```python
from build123d import *

# Parameters (mm, degrees)
SKETCH1_W           = 154.5
SKETCH1_H           = 74.4
BOSS_EXTRUDE1_DEPTH = 7.4
FILLET1_R           = 10
CHAMFER1_SIZE       = 1
FILLET2_R           = 2
SKETCH2_R           = 4.3
BOSS_EXTRUDE2_DEPTH = 0.6
CHAMFER2_SIZE       = 0.3
CUT_EXTRUDE1_DEPTH  = 6.75


with BuildPart() as part:
    # Sketch1 → Boss-Extrude1 (new body)
    with BuildSketch(Plane(origin=(0, 0, 0), x_dir=(1, 0, 0), z_dir=(0, 1, 0))):
        Rectangle(SKETCH1_W, SKETCH1_H)
    extrude(amount=BOSS_EXTRUDE1_DEPTH)

    # Fillet1
    fillet1_edges = [part.edges().sort_by_distance(p)[0] for p in [
        (77.25, 3.7, 37.2),
        (-77.25, 3.7, 37.2),
        (-77.25, 3.7, -37.2),
        (77.25, 3.7, -37.2),
    ]]
    fillet(fillet1_edges, radius=FILLET1_R)

    # Chamfer1
    chamfer1_edges = [part.edges().sort_by_distance(p)[0] for p in [
        (-77.25, 7.4, 0),
        (0, 7.4, -37.2),
        (77.25, 7.4, 0),
        (0, 7.4, 37.2),
        (74.321067812, 7.4, 34.271067812),
        (-74.321067812, 7.4, 34.271067812),
        (74.321067812, 7.4, -34.271067812),
        (-74.321067812, 7.4, -34.271067812),
    ]]
    chamfer(chamfer1_edges, length=CHAMFER1_SIZE)

    # Fillet2
    fillet2_edges = [part.edges().sort_by_distance(p)[0] for p in [
        (-77.25, 0, 0),
        (77.25, 0, 0),
        (0, 0, 37.2),
        (0, 0, -37.2),
        (74.321067812, 0, 34.271067812),
        (-74.321067812, 0, 34.271067812),
        (74.321067812, 0, -34.271067812),
        (-74.321067812, 0, -34.271067812),
    ]]
    fillet(fillet2_edges, radius=FILLET2_R)

    # Sketch2 → Boss-Extrude2 (add)
    with BuildSketch(Plane.XZ):
        with Locations((-68.95, -13.75)):
            Circle(SKETCH2_R)
        with BuildLine():
            Line((-73.25, -13.75), (-73.25, -23.65))
            ThreePointArc((-73.25, -23.65), (-68.95, -19.35), (-64.65, -23.65))
            Line((-64.65, -23.65), (-64.65, -13.75))
            ThreePointArc((-64.65, -13.75), (-68.95, -18.05), (-73.25, -13.75))
        make_face()
        with Locations((-68.95, -23.65)):
            Circle(SKETCH2_R)
    extrude(amount=BOSS_EXTRUDE2_DEPTH)

    # Chamfer2
    chamfer2_edges = [part.edges().sort_by_distance(p)[0] for p in [
        (-64.65, -0.6, -18.7),
        (-73.25, -0.6, -18.7),
        (-68.95, -0.6, -9.45),
        (-68.95, -0.6, -27.95),
    ]]
    chamfer(chamfer2_edges, length=CHAMFER2_SIZE)

    # Sketch3 → Cut-Extrude1 (cut)
    with BuildSketch(Plane(origin=(77.25, 0, 0), x_dir=(0, 0, -1), z_dir=(1, 0, 0))):
        with BuildLine():
            Line((-2.9, 4.8), (2.9, 4.8))
            ThreePointArc((2.9, 4.8), (4.2, 3.5), (2.9, 2.2))
            Line((2.9, 2.2), (-2.9, 2.2))
            ThreePointArc((-2.9, 2.2), (-4.2, 3.5), (-2.9, 4.8))
        make_face()
    extrude(amount=-CUT_EXTRUDE1_DEPTH, mode=Mode.SUBTRACT)


solid = part.part
```
The listing builds one solid part. Answer for the finished solid, in the listing's coordinates (mm). A direction names the side the tool comes from. Give positions to 0.01 mm unless a question says otherwise; leave off trailing zeros. Order: outer loops, then holes, each group sorted by start corner. A loop starts at its lowest first (then second) coordinate and runs counter-clockwise, first axis right, second up. Notation, with made-up numbers: (10.25, 53) -> (57.25, 53) arc R18 ccw to (57.25, 79) -> close; hole circle Ø11 at (-24.75, 56). An arc over 180 degrees is marked (long way). Answer as a JSON object with one key per item and string values. Group by question number.
Item 1: A tool of negligible diameter and unlimited length cuts with its end or side. For faces 4 (the flat face through (70.5, 4, 0)), 5 (the conical face through (-73.798, 7.24, -33.605)), from which of +Z, -Z, +X, -X, +Y, -Y can it reach the whole face along a straight path? Write none if from no direction.
Item 2: The part is cut by section B-B on x = -31.5. Write down the section's boundary in (y, z).
Item 3: The part is cut by section A-A on z = -21. Write down the section's boundary in (x, y).
Item 4: Flat-ended cylindrical pins translate along their axes: pin 1 (8 mm diameter, centred on x = 52.5, z = -29.5, fed in from -Y); pin 2 (2 mm diameter, centred on y = 3, z = 0, fed in from +X). Find the tip coordinate at first contact, or state that the pin passes through.
Item 5: Determine the mould class of faces 1 (the cylindrical face through (74.24, 4.23, 34.35)), 2 (the cylindrical face through (73.9, 3.5, -4.2)), 3 (the flat face through (-1, 7.4, -1)) for opening direction Z: pulls with the +Z half, pulls with the -Z half, needs draft (parallel to the pull), parting line crosses it, or undercut.
Item 6: Consider L1, parallel to Y at x = -9, z = -27.5; L2, parallel to X at y = 2.5, z = 27.5; L3, parallel to Z at x = -57, y = 1.25. Determine where each line is inside the solid, lowest interval first. Write a range as from..to.
Result set:
{
 "1": {"face 4": "+X", "face 5": "-Z, -X, +Y"},
 "2": {"outline": "(0, -35.2) arc R2 ccw to (2, -37.2) -> (6.4, -37.2) -> (7.4, -36.2) -> (7.4, 36.2) -> (6.4, 37.2) -> (2, 37.2) arc R2 ccw to (0, 35.2) -> close"},
 "3": {"outline": "(-77.25, 2) arc R2 ccw to (-75.25, 0) -> (-73.25, 0) -> (-73.25, -0.3) -> (-72.95, -0.6) -> (-64.95, -0.6) -> (-64.65, -0.3) -> (-64.65, 0) -> (75.25, 0) arc R2 ccw to (77.25, 2) -> (77.25, 6.4) -> (76.25, 7.4) -> (-76.25, 7.4) -> (-77.25, 6.4) -> close"},
 "4": {"pin 1": "y = 0", "pin 2": "x = 77.25"},
 "5": {"face 1": "pulls with the +Z half", "face 2": "undercut", "face 3": "needs draft"},
 "6": {"L1": "0..7.4", "L2": "-77.25..77.25", "L3": "-37.05..37.05"}
}
